from build123d import *

# Parameters (mm, degrees)
SKETCH1_R      = 3.175
EXTRUDE1_DEPTH = 25.4
CHAMFER1_SIZE  = 0.635
EXTRUDE7_DEPTH = 26.4


with BuildPart() as part:
    # Sketch1 → Extrude1 (new body, symmetric)
    with BuildSketch(Plane.XY):
        Circle(SKETCH1_R)
    extrude(amount=EXTRUDE1_DEPTH, both=True)

    # Chamfer1
    chamfer1_edges = [part.edges().sort_by_distance(p)[0] for p in [
        (-3.175, 0, -25.4),
        (-3.175, 0, 25.4),
    ]]
    chamfer(chamfer1_edges, length=CHAMFER1_SIZE)

    # Sketch13 → Extrude7 (cut, through all)
    with BuildSketch(Plane.XY):
        with BuildLine():
            Line((-1.5875, 2.749630657), (1.5875, 2.749630657))
            ThreePointArc((1.5875, 2.749630657), (0, 3.175), (-1.5875, 2.749630657))
        make_face()
    extrude(amount=EXTRUDE7_DEPTH, mode=Mode.SUBTRACT)


solid = part.part
Input: part model. Units: mm. Frame: model coordinates. A direction names the side the tool comes from. Give positions to 0.01 mm unless a question says otherwise; leave off trailing zeros. Loops run counter-clockwise (first coordinate to the right, second up) from the corner with the lowest first, then second, coordinate; pieces in that order, holes last. Notation, with made-up numbers: (-0.5, 76) -> (57.5, 76) arc R25 cw to (57.5, 93) -> close; hole circle Ø7 at (-19, 15.25). An arc over 180 degrees is marked (long way). Answer as a JSON object with one key per item and string values. Group by question number.
Item 1: Reachability of faces 1 (the flat face through (0, 0, 25.4)), 2 (the flat face through (0, 2.75, 12)) from +Z, -Z, +X, -X, +Y, -Y: full face, straight path, thin tool, end or side. Return the list, or none.
Item 2: Pin query (flat end, axial travel): P1, Ø1.5, axis at x = -1, z = -20, coming from the +Y side; P2, Ø1, axis at x = 0.5, z = 8.5, coming from the +Y side; P3, Ø1, axis at y = 1, z = -13.5, coming from the +X side. Return the tip coordinate at first contact, or that it passes through.
Item 3: Line query: probe 1 along Y at (x, z) = (2.75, 17); probe 2 along X at (y, z) = (2.25, 10.5); probe 3 along X at (y, z) = (-2.5, 0). Output: solid intervals per line, ascending.
Item 4: Cut plane C-C, the plane z = -21.5. Return the cut outline in (x, y) (3 decimals).
Item 5: Cut plane A-A, the plane x = 0. Return the cut outline in (y, z) (3 decimals).
Checks:
{
 "1": {"face 1": "+Z, +X, -X, +Y, -Y", "face 2": "+Z, +X, -X, +Y"},
 "2": {"P1": "stops at y = 3.17", "P2": "stops at y = 2.75", "P3": "stops at x = 3.14"},
 "3": {"probe 1": "y = -1.59 to 1.59", "probe 2": "x = -2.24 to 2.24", "probe 3": "x = -1.96 to 1.96"},
 "4": {"outline": "circle Ø6.35 at (0, 0)"},
 "5": {"outline": "(-3.175, -24.765) -> (-2.54, -25.4) -> (2.54, -25.4) -> (3.175, -24.765) -> (3.175, 0) -> (2.75, 0) -> (2.75, 25.19) -> (2.54, 25.4) -> (-2.54, 25.4) -> (-3.175, 24.765) -> close"}
}
